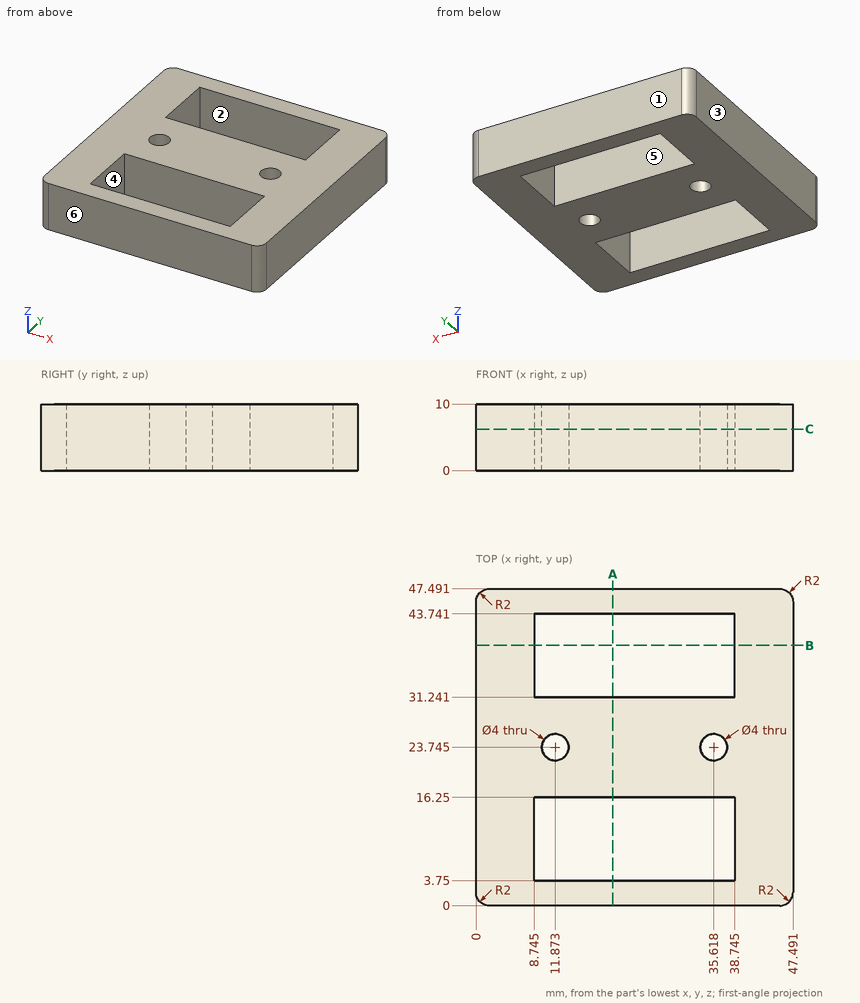
Print and shaded views of the part. All mm, measured from the part's lowest x, y and z. A direction names the side the tool comes from. Coordinates: 2 decimals unless noted, no trailing zeros. Order: outer loops, then holes, each group sorted by start corner. A loop starts at its lowest first (then second) coordinate and runs counter-clockwise, first axis right, second up. Notation, with made-up numbers: (33, 19.25) - (46, 19.25) arc R22 ccw to (46, 58.25) - close; hole circle Ø2 at (55, 39.25). An arc over 180 degrees is marked (long way). Return JSON: item names as keys, results as strings. Group by question number.
Item 1: Pull direction Y, two halves, no side cores. Call the marked faces 1, 2, 3 and 4: pulls with the +Y half, pulls with the -Y half, needs draft (parallel to the pull), parting line crosses it, or undercut.
Item 2: Cut at C-C (z = 6.25). State how many separate pieces and enclosed holes the cut face has, plus the area to 3 significant figures.
Item 3: Drill centre lines: probe 1 along Y at (x, z) = (26.5, 8.75); probe 2 along X at (y, z) = (33, 3.25) (1 decimal); probe 3 along Y at (x, z) = (12, 5.5). Where is each one in solid material? Low to high. Write a range as from..to.
Item 4: Which spindle directions (+Z, -Z, +X, -X, +Y, -Y) get a long thin tool onto all of the face, cutting with end or side? Do the marked faces 5 and 6. Say none if no direction does.
Item 5: Cut at B-B (y = 39). List the corners of the cut face in (x, z) (1 decimal), plus the area to 3 significant figures.
Item 6: Cut at A-A (x = 20.5). List the corners of the cut face in (y, z).
Item 7: Pin check, flat tip, straight feed: pin 1 (3.5 mm diameter, centred on x = 11.87, y = 23.75, fed in from +Z). Stop position of the tip, or through.
Check values:
{
 "1": {"face 1": "pulls with the +Y half", "face 2": "undercut", "face 3": "needs draft", "face 4": "undercut"},
 "2": {"separate pieces": "1", "enclosed holes": "4", "area": "1,480 mm2"},
 "3": {"probe 1": "y = 0..3.75, 16.25..31.24, 43.74..47.49", "probe 2": "x = 0..8.7, 38.7..47.5", "probe 3": "y = 0..3.75, 16.25..21.75, 25.74..31.24, 43.74..47.49"},
 "4": {"face 5": "+Z, -Z", "face 6": "+Z, -Z, +X, -X, -Y"},
 "5": {"outline": "(0, 0) - (8.7, 0) - (8.7, 10) - (0, 10) - close; (38.7, 0) - (47.5, 0) - (47.5, 10) - (38.7, 10) - close", "area": "175 mm2"},
 "6": {"outline": "(0, 0) - (3.75, 0) - (3.75, 10) - (0, 10) - close; (16.25, 0) - (31.24, 0) - (31.24, 10) - (16.25, 10) - close; (43.74, 0) - (47.49, 0) - (47.49, 10) - (43.74, 10) - close"},
 "7": {"pin 1": "passes through"}
}
